Check sheet for the modelled part. Datum: model origin and axes. Units: mm. Face numbers are marked on the shaded views. A direction names the side the tool comes from. Coordinates: 2 decimals unless noted, no trailing zeros. One line per item, written item: value. Start each with the question number.
1) Scan lines: line 1 along Y through (x, z) = (5.5, 17); line 2 along Z through (x, y) = (5, -3); line 3 along Z through (x, y) = (14.5, 5.5). Record each from-to range of solid material in increasing order. Write a range as [from, to].
2) Set-up check for the marked faces 1 and 2: record each of +Z, -Z, +X, -X, +Y, -Y from which the full face is reachable in a straight line by a thin tool's end or side.
3) Gauge pin test, flat ends, axial feed: P1, Ø3, axis at x = 1, z = 7.5, coming from the +Y side; P2, Ø3, axis at y = -3, z = 14.5, coming from the -X side; P3, Ø6, axis at x = 9, z = 13.5, coming from the -Y side. Record the tip position at first contact, or that the pin passes through.
```python
from build123d import *

# Parameters (mm, degrees)
F2_R = 0.713231
F3_R = 5.459817


with BuildPart() as f1:
    # F0 (on Front) → F1 (revolve)
    with BuildSketch(Plane.XZ):
        Polygon((0, 19.496445), (0, 0), (2.556912, 0), (2.556912, 5.007284), (16.619919, 19.496445), align=None)
    revolve(axis=Axis((0, 0, 9.748222), (0, 0, -1)))

    # F2
    f2_edges = [f1.edges().sort_by_distance(p)[0] for p in [
        (-16.619919, 0, 19.496445),
    ]]
    fillet(f2_edges, radius=F2_R)

    # F3
    f3_edges = [f1.edges().sort_by_distance(p)[0] for p in [
        (-2.556912, 0, 5.007284),
    ]]
    fillet(f3_edges, radius=F3_R)


solid = f1.part
```
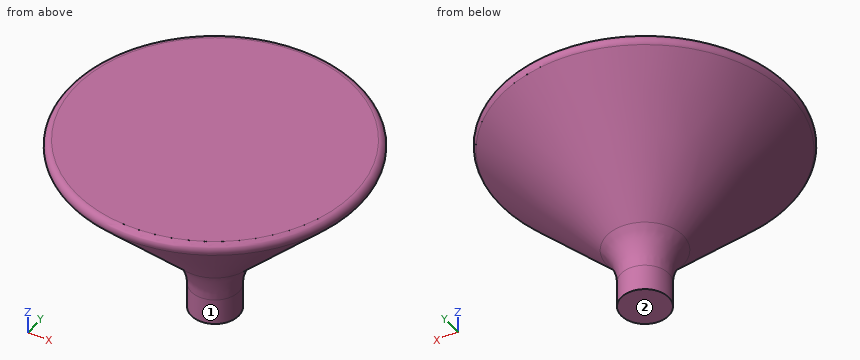
Answers:
1. line 1: y = [-13.09, 13.09]
1. line 2: z = [8.38, 19.5]
1. line 3: z = [18.36, 19.21]
2. face 1: -Z
2. face 2: -Z, +X, -X, +Y, -Y
3. P1: stops at y = 6.37
3. P2: stops at x = -12.92
3. P3: stops at y = -11.01
